from build123d import *

# Parameters (mm, degrees)
SKETCH2_R           = 41
BOSS_EXTRUDE1_DEPTH = 40
HOME_DEPTH          = 9
END_R_DEPTH         = 9
END_L_DEPTH         = 10
SKETCH8_R           = 35
CUT_EXTRUDE1_DEPTH  = 10
CUT_EXTRUDE3_DEPTH  = 25
CUT_EXTRUDE4_REACH  = 7
SKETCH11_R          = 3.1
SKETCH12_R          = 6
CUT_EXTRUDE5_DEPTH  = 1


with BuildPart() as part:
    # Sketch2 → Boss-Extrude1 (new body)
    with BuildSketch(Plane(origin=(0, 0, 0), x_dir=(1, 0, 0), z_dir=(0, 1, 0))):
        Circle(SKETCH2_R)
    extrude(amount=BOSS_EXTRUDE1_DEPTH)

    # Sketch3 → Home (add)
    with BuildSketch(Plane(origin=(0, 0, 0), x_dir=(1, 0, 0), z_dir=(0, 1, 0))):
        with BuildLine():
            ThreePointArc((28.604048631, -34.088977719), (29.776311983, -33.069944734), (30.912297485, -32.010621115))
            ThreePointArc((30.912297485, -32.010621115), (32.604689255, -28.381998607), (32.953955321, -24.393376738))
            ThreePointArc((32.953955321, -24.393376738), (27.434354861, -30.468937845), (20.815120959, -35.323232291))
            ThreePointArc((20.815120959, -35.323232291), (24.818400986, -35.392804054), (28.604048631, -34.088977719))
        make_face()
    extrude(amount=HOME_DEPTH)

    # Sketch4 → End R (add)
    with BuildSketch(Plane(origin=(0, 10, 0), x_dir=(1, 0, 0), z_dir=(0, 1, 0))):
        with BuildLine():
            Line((41.259681528, -16.669993407), (39.164522306, -12.130135718))
            ThreePointArc((39.164522306, -12.130135718), (34.826898772, -21.635321166), (28.227629104, -29.735516729))
            ThreePointArc((28.227629104, -29.735516729), (32.143955565, -28.90276331), (35.539280197, -26.78076853))
            ThreePointArc((35.539280197, -26.78076853), (38.730828469, -21.912848425), (41.259681528, -16.669993407))
        make_face()
    extrude(amount=END_R_DEPTH)

    # Sketch6 → End L (add)
    with BuildSketch(Plane(origin=(0, 19, 0), x_dir=(1, 0, 0), z_dir=(0, 1, 0))):
        with BuildLine():
            Line((-41.259681528, -16.669993407), (-39.304086987, -11.669993407))
            ThreePointArc((-39.304086987, -11.669993407), (-34.902749486, -21.512742231), (-28.087672455, -29.867752779))
            ThreePointArc((-28.087672455, -29.867752779), (-32.085635632, -28.981220402), (-35.539280197, -26.78076853))
            ThreePointArc((-35.539280197, -26.78076853), (-38.730828469, -21.912848425), (-41.259681528, -16.669993407))
        make_face()
    extrude(amount=END_L_DEPTH)

    # Sketch8 → Cut-Extrude1 (cut)
    with BuildSketch(Plane.XZ):
        Circle(SKETCH8_R)
    extrude(amount=-CUT_EXTRUDE1_DEPTH, mode=Mode.SUBTRACT)

    # Sketch10 → Cut-Extrude3 (cut)
    with BuildSketch(Plane.XZ.offset(-10)):
        with BuildLine():
            Line((-2.5, -8.259618977), (2.5, -8.259618977))
            ThreePointArc((2.5, -8.259618977), (2.853553391, -8.406065586), (3, -8.759618977))
            Line((3, -8.759618977), (3, -10.842624221))
            ThreePointArc((3, -10.842624221), (0, 11.25), (-3, -10.842624221))
            Line((-3, -10.842624221), (-3, -8.759618977))
            ThreePointArc((-3, -8.759618977), (-2.853553391, -8.406065586), (-2.5, -8.259618977))
        make_face()
    extrude(amount=-CUT_EXTRUDE3_DEPTH, mode=Mode.SUBTRACT)

    # Sketch11 → Cut-Extrude4 (cut, up to next)
    with BuildSketch(Plane.XZ.offset(-35), mode=Mode.PRIVATE) as cut_extrude4_sk1:
        Circle(SKETCH11_R)
    cut_extrude4_tool1 = extrude(cut_extrude4_sk1.sketch, amount=-CUT_EXTRUDE4_REACH, mode=Mode.PRIVATE) & part.part
    add(cut_extrude4_tool1.solids().sort_by_distance((0, 35, 0))[0], mode=Mode.SUBTRACT)

    # Sketch12 → Cut-Extrude5 (cut)
    with BuildSketch(Plane(origin=(0, 40, 0), x_dir=(1, 0, 0), z_dir=(0, 1, 0))):
        Circle(SKETCH12_R)
    extrude(amount=-CUT_EXTRUDE5_DEPTH, mode=Mode.SUBTRACT)


solid = part.part
Could you check a few things on this model? Use its own coordinates, in mm. A direction names the side the tool comes from. Give positions to 0.01 mm unless a question says otherwise; leave off trailing zeros. Loops run counter-clockwise (first coordinate to the right, second up) from the corner with the lowest first, then second, coordinate; pieces in that order, holes last. Notation, with made-up numbers: (10, 21) -> (43, 21) arc R28 ccw to (43, 57) -> close; hole circle Ø10 at (21.25, 79). An arc over 180 degrees is marked (long way). Return JSON: item names as keys, results as strings.
Item 1: If we section it at C-C on y = 11.5: List the corners of the cut face in (x, z) for me, plus the area to 3 significant figures.
Geometry results:
{"outline": "(28.23, 29.74) arc R41 ccw (long way) to (39.16, 12.13) -> (41.26, 16.67) arc R44.5 ccw to (35.54, 26.78) arc R11.53 ccw to start; hole (-3, -10.84) -> (-3, -8.76) arc R0.5 cw to (-2.5, -8.26) -> (2.5, -8.26) arc R0.5 cw to (3, -8.76) -> (3, -10.84) arc R11.25 ccw (long way) to start", "area": "4,960 mm²"}
Item 2: If we section it at B-B on z = 0: List the corners of the cut face in (x, y) for me.
Geometry results:
{"outline": "(-41, 0) -> (-35, 0) -> (-35, 10) -> (-11.25, 10) -> (-11.25, 35) -> (-3.1, 35) -> (-3.1, 39) -> (-6, 39) -> (-6, 40) -> (-41, 40) -> close; (3.1, 35) -> (11.25, 35) -> (11.25, 10) -> (35, 10) -> (35, 0) -> (41, 0) -> (41, 40) -> (6, 40) -> (6, 39) -> (3.1, 39) -> close"}
Item 3: I need wall thicknesses on L1, parallel to X at y = 25, z = 0; L2, parallel to X at y = 39.6, z = 0; L3, parallel to Y at x = 2, z = -26. Which ranges of each line are inside material? Lowest first, please. Write a range as from..to.
Geometry results:
{"L1": "x = -41..-11.25, 11.25..41", "L2": "x = -41..-6, 6..41", "L3": "y = 10..40"}
Item 4: If we section it at A-A on x = 0: List the corners of the cut face in (y, z) for me, plus the area to 3 significant figures.
Geometry results:
{"outline": "(0, -41) -> (40, -41) -> (40, -6) -> (39, -6) -> (39, -3.1) -> (35, -3.1) -> (35, -8.26) -> (10, -8.26) -> (10, -35) -> (0, -35) -> close; (0, 35) -> (10, 35) -> (10, 11.25) -> (35, 11.25) -> (35, 3.1) -> (39, 3.1) -> (39, 6) -> (40, 6) -> (40, 41) -> (0, 41) -> close", "area": "2,060 mm²"}
Item 5: We'd pull the mould along Z, two halves only. Please class faces 1 (the cylindrical face through (24.76, 4.44, 35.4)), 2 (the flat face through (3, 22, -10)), 3 (the flat face through (36, 19, 22)): +Z half, -Z half, draft (parallel to the pull), parting line (faces both ways), or undercut.
Geometry results:
{"face 1": "+Z half", "face 2": "undercut", "face 3": "draft"}
Item 6: If we section it at D-D on y = 34: List the corners of the cut face in (x, z) for me.
Geometry results:
{"outline": "circle Ø82 at (0, 0); hole (-3, -10.84) -> (-3, -8.76) arc R0.5 cw to (-2.5, -8.26) -> (2.5, -8.26) arc R0.5 cw to (3, -8.76) -> (3, -10.84) arc R11.25 ccw (long way) to start"}
Item 7: I'm going to push flat-ended pins straight in: pin 1 (11 mm diameter, centred on x = 0, z = 0, fed in from +Y); pin 2 (2.5 mm diameter, centred on y = 25.5, z = -10.5, fed in from -X); pin 3 (1 mm diameter, centred on x = -24.5, y = 19.5, fed in from +Z). Where does each tip first touch, or does it pass through?
Geometry results:
{"pin 1": "stops at y = 39", "pin 2": "stops at x = -39.94", "pin 3": "stops at z = 33.24"}
Item 8: Which directions (+Z, -Z, +X, -X, +Y, -Y) give clear straight access to the entire face, cutting with the end or side of a thin tool? Please do faces 4 (the flat face through (40.227, 14.437, 14.432)), 5 (the flat face through (28, 9, 31)), 6 (the flat face through (-8.3, 10, 8.3)).
Geometry results:
{"face 4": "+X, +Y, -Y", "face 5": "+Z, +X", "face 6": "-Y"}
